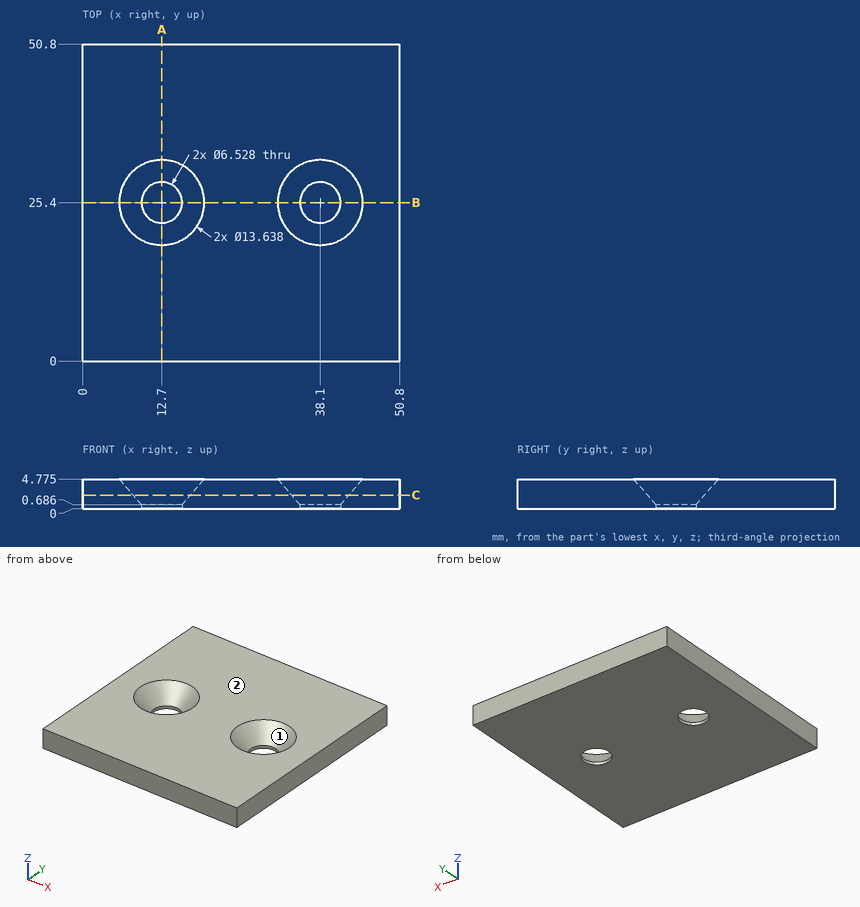
Design review of the part shown in the three views and the two pictorial views. Dimensions are in mm from the part's minimum x, y and z. Round coordinates to 2 decimals unless told otherwise and drop trailing zeros. Loops run counter-clockwise (first coordinate to the right, second up) from the corner with the lowest first, then second, coordinate; pieces in that order, holes last.
1) The part is to be moulded in two halves that separate along X. For the marked faces 1 and 2, say which applies: pulls with the +X half, pulls with the -X half, needs draft (parallel to the pull), parting line crosses it, or undercut.
Values follow:
face 1: undercut
face 2: needs draft
2) Clearance check with a flat-ended pin moving along its axis: P1, Ø8, axis at x = 17, y = 36.5, coming from the -Z side. State where the tip first meets the part, or that it passes through.
Values follow:
P1: stops at z = 0
3) Consider section A-A on x = 12.7. State the section outline as (y, z) points (1 decimal).
Values follow:
outline: (0, 0) - (22.1, 0) - (22.1, 0.7) - (18.6, 4.8) - (0, 4.8) - close; (28.7, 0) - (50.8, 0) - (50.8, 4.8) - (32.2, 4.8) - (28.7, 0.7) - close
4) Wall thickness on line 1 along Y through (x, z) = (38.1, 0.5); line 2 along X through (y, z) = (27.5, 4.15) (1 decimal); line 3 along X through (y, z) = (27, 1.95): over which ranges is each line inside the solid? List them lowest first.
Values follow:
line 1: y = 0 to 22.14, 28.66 to 50.8
line 2: x = 0 to 6.8, 18.6 to 32.2, 44 to 50.8
line 3: x = 0 to 8.64, 16.76 to 34.04, 42.16 to 50.8
5) Consider section B-B on y = 25.4. Give the number of separate pieces and of enclosed holes in the cut face, then the cut area to 3 significant figures.
Values follow:
separate pieces: 3
enclosed holes: 0
area: 151 mm2
6) Consider section C-C on z = 2.2. State the section outline as (x, y) points.
Values follow:
outline: (0, 0) - (50.8, 0) - (50.8, 50.8) - (0, 50.8) - close; hole circle Ø9.16 at (12.7, 25.4); hole circle Ø9.16 at (38.1, 25.4)
